The listing builds one solid part. Answer for the finished solid, in the listing's coordinates (mm). A direction names the side the tool comes from. Round coordinates to 2 decimals unless told otherwise and drop trailing zeros. Write each loop counter-clockwise with the first axis right and the second up, starting at its lowest first coordinate (ties: lowest second). Pieces come first, ordered by that corner, then holes. Notation, with made-up numbers: M -12.75,81 L -8.75,81 A29 ccw -8.75,106 Z; hole C 78,88 d5. An arc over 180 degrees is marked long. Write each question's results on one line, items separated by ' | '.
from build123d import *

# Parameters (mm, degrees)
F1_DEPTH = 11.7
F3_DEPTH = 14
F4_R     = 2.7
F5_DEPTH = 11.5
F6_SIZE  = 0.5
F7_W     = 10
F7_H     = 10
F8_DEPTH = 5


with BuildPart() as f1:
    # F0 (on Top) → F1 (new body)
    with BuildSketch(Plane.XY):
        Polygon((0, 4.8), (0, 0), (0, -4.8), (12.6, -7), (21.6, -7), (21.6, 0), (21.6, 7), (12.6, 7), align=None)
    extrude(amount=F1_DEPTH)

    # F2 (on face) → F3 (cut, through all)
    with BuildSketch(Plane.XZ.offset(7)):
        Polygon((0, 10.45), (12.6, 11.7), (0, 11.7), align=None)
        Polygon((0, 0), (12.6, 0), (0, 1.25), align=None)
    extrude(amount=-F3_DEPTH, mode=Mode.SUBTRACT)

    # F4 (on face) → F5 (join)
    with BuildSketch(Plane(origin=(0, 0, 0), x_dir=(0, -1, 0), z_dir=(-1, 0, 0))):
        with Locations((0, 5.85)):
            Circle(F4_R)
    extrude(amount=F5_DEPTH)

    # F6
    f6_edges = [f1.edges().sort_by_distance(p)[0] for p in [
        (-11.5, 2.7, 5.85),
    ]]
    chamfer(f6_edges, length=F6_SIZE)

    # F7 (on face) → F8 (join)
    with BuildSketch(Plane.YZ.offset(21.6)):
        with Locations((0, 7.9)):
            Rectangle(F7_W, F7_H)
    extrude(amount=F8_DEPTH)


solid = f1.part
1) Find the intervals of material crossed by line 1 (X direction, y = -4.5, z = 10); line 2 (Z direction, x = 18.5, y = -5.5); line 3 (X direction, y = -4.5, z = 12), in increasing order.
Return value:
line 1: 0 to 26.6 | line 2: 0 to 11.7 | line 3: 21.6 to 26.6
2) Section C-C (y = -3.25) is taken. Determine the outline of the cut face in (x, z).
Return value:
outline: M 0,1.25 L 12.6,0 L 21.6,0 L 21.6,2.9 L 26.6,2.9 L 26.6,12.9 L 21.6,12.9 L 21.6,11.7 L 12.6,11.7 L 0,10.45 Z
3) Section A-A (y = 0) is taken. Determine the outline of the cut face in (x, z), then the cut area to 3 significant figures.
Return value:
outline: M -11.5,3.65 L -11,3.15 L 0,3.15 L 0,1.25 L 12.6,0 L 21.6,0 L 21.6,2.9 L 26.6,2.9 L 26.6,12.9 L 21.6,12.9 L 21.6,11.7 L 12.6,11.7 L 0,10.45 L 0,8.55 L -11,8.55 L -11.5,8.05 Z | area: 349 mm²
4) Section D-D (z = 5.85) is taken. Determine the outline of the cut face in (x, y), then the cut area to 3 significant figures.
Return value:
outline: M -11.5,-2.2 L -11,-2.7 L 0,-2.7 L 0,-4.8 L 12.6,-7 L 21.6,-7 L 21.6,-5 L 26.6,-5 L 26.6,5 L 21.6,5 L 21.6,7 L 12.6,7 L 0,4.8 L 0,2.7 L -11,2.7 L -11.5,2.2 Z | area: 387 mm²
5) Each of these flat-tipped pins is pushed along its axis until it touches: pin 1 (4 mm diameter, centred on y = -3, z = 2, fed in from -X); pin 2 (5 mm diameter, centred on x = -5.5, z = 5, fed in from +Y); pin 3 (6 mm diameter, centred on x = 6, y = -3, fed in from -Z). Where does it stop, or does it pass through?
Return value:
pin 1: x = 0 | pin 2: y = 2.7 | pin 3: z = 0.36
6) Section B-B (z = 10) is taken. Determine the outline of the cut face in (x, y), then the cut area to 3 significant figures.
Return value:
outline: M 0,-4.8 L 12.6,-7 L 21.6,-7 L 21.6,-5 L 26.6,-5 L 26.6,5 L 21.6,5 L 21.6,7 L 12.6,7 L 0,4.8 Z | area: 325 mm²
7) A tool of negligible diameter and unlimited length cuts with its end or side. For faces 1 (the face through (0, 2, 8)), 2 (the face through (17, 0, 11.7)), 3 (the face through (24, 0, 2.9)), 4 (the face through (24, 5, 8)), 5 (the face through (24, -5, 8)), from which of +Z, -Z, +X, -X, +Y, -Y can it reach the whole face along a straight path? Write none if from no direction.
Return value:
face 1: -X | face 2: +Z, -X, +Y, -Y | face 3: -Z, +X, +Y, -Y | face 4: +Z, -Z, +X, +Y | face 5: +Z, -Z, +X, -Y
